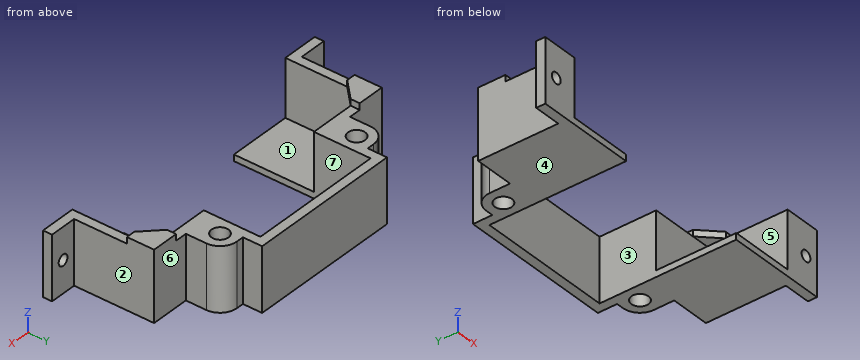
Autodesk Inventor part; units mm, degrees
ref_plane "YZ Plane" through (0, 0, 0) normal (1, 0, 0) x (0, 1, 0)
ref_plane "XZ Plane" through (0, 0, 0) normal (0, 1, 0) x (-1, 0, 0)
ref_plane "XY Plane" through (0, 0, 0) normal (0, 0, 1) x (1, 0, 0)
sketch "スケッチ1" plane through (0, 0, 0) normal (0, 0, 1) x (1, 0, 0)
  line L0 (0, 0) -> (0, 17.65)
  line L1 (0, 17.65) -> (28, 17.65)
  line L2 (28, 17.65) -> (28, 30.15)
  line L3 (28, 30.15) -> (58, 30.15)
  line L4 (58, 30.15) -> (58, 0)
  line L5 (58, 0) -> (60, 0)
  line L6 (60, 0) -> (60, 32.15)
  line L7 (60, 32.15) -> (28, 32.15)
  line L8 (28, 32.15) -> (26, 32.15)
  line L9 (26, 32.15) -> (26, 19.65)
  line L10 (26, 19.65) -> (-2, 19.65)
  line L11 (-2, 19.65) -> (-2, 0)
  line L12 (-2, 0) -> (0, 0)
  dimension "d0" = 17.65
  dimension "d1" = 28
  dimension "d2" = 12.5
  dimension "d3" = 30
  dimension "d4" = 2
  dimension "d5" = 32.15
  dimension "d6" = 32
  dimension "d7" = 2
  dimension "d8" = 12.5
  dimension "d9" = 28
extrude "押し出し1" add sketch "スケッチ1" along normal blind 14
sketch "スケッチ2" plane through (60, 0, 0) normal (1, 0, 0) x (0, 0, -1)
  line L0 (0, 0) -> (-14, 0)
  line L1 (-14, 0) -> (0, 0)
  line L2 (0, 0) -> (0, 2)
  line L3 (0, 2) -> (-14, 2)
  line L4 (-14, 2) -> (-14, 0)
  dimension "d12" = 14
  dimension "d13" = 2
extrude "押し出し2" add sketch "スケッチ2" along normal blind 7
sketch "スケッチ3" plane through (-2, 0, 0) normal (-1, 0, 0) x (0, 0, 1)
  line L0 (14, 2) -> (0, 2)
  line L1 (0, 0) -> (14, 0)
  line L2 (14, 0) -> (14, 2)
  line L3 (14, 2) -> (0, 2)
  line L4 (0, 2) -> (0, 0)
  dimension "d16" = 14
extrude "押し出し3" add sketch "スケッチ3" along normal blind 7
sketch "スケッチ4" plane through (0, 0, 14) normal (0, 0, 1) x (1, 0, 0)
  line L0 (60, 32.15) -> (60, 24.15)
  line L1 (60, 24.15) -> (61.6, 24.15)
  arc A0 (61.6, 20.4) -> (61.6, 27.9) centre (61.6, 24.15) ccw
  line L2 (61.6, 24.15) -> (61.6, 20.4) construction
  line L3 (61.6, 24.15) -> (61.6, 27.9) construction
  line L4 (61.6, 27.9) -> (60, 27.9)
  line L5 (61.6, 20.4) -> (60, 20.4)
  line L6 (60, 2) -> (60, 32.15)
  line L7 (60, 27.9) -> (60, 20.4)
  point P0 (0, 0)
  dimension "d47" = 8
  dimension "d48" = 1.6
  dimension "d49" = 3.75
  dimension "d50" = 180
extrude "押し出し4" add sketch "スケッチ4" against normal blind 14
hole "穴3" at (61.6, 24.15, 14) direction (0, 0, -1) diameter 3.75 end through all
sketch "スケッチ7" plane through (0, 0, 14) normal (0, 0, 1) x (1, 0, 0)
  line L0 (60, 32.15) -> (26, 32.15)
  line L1 (26, 32.15) -> (26, 24.15)
  line L2 (26, 24.15) -> (24.4, 24.15)
  arc A0 (24.4, 27.9) -> (24.4, 20.4) centre (24.4, 24.15) ccw
  line L3 (24.4, 27.9) -> (26, 27.9)
  line L4 (24.4, 20.4) -> (26, 20.4)
  line L5 (26, 20.4) -> (26, 27.9)
  line L6 (26, 32.15) -> (26, 19.65)
  circle A1 centre (24.4, 24.15) radius 1.875
  point P0 (0, 0)
  dimension "d60" = 8
  dimension "d61" = 1.6
  dimension "d62" = 3.75
  dimension "d63" = 3.75
extrude "押し出し6" add sketch "スケッチ7" against normal blind 14 contours L1 A1 L5 L4 A0 L3 | L1 L5 A1 picked at (23.6929, 24.15)
hole "穴4" at (24.4, 24.15, 14) direction (0, 0, -1) diameter 3.75 end through all
sketch "スケッチ10" plane through (0, 17.65, 0) normal (0, -1, 0) x (1, 0, 0)
  line L0 (28, 14) -> (58, 14)
  line L1 (0, 0) -> (28, 0)
  line L2 (28, 0) -> (28, 14)
  line L3 (28, 14) -> (0, 14)
  line L4 (0, 14) -> (0, 0)
extrude "押し出し7" cut sketch "スケッチ10" against normal blind 0.6
sketch "スケッチ11" plane through (0, 0, 0) normal (0, -1, 0) x (1, 0, 0)
  line L0 (0, 14) -> (-9, 14)
  line L1 (60, 0) -> (67, 0)
  line L2 (-9, 14) -> (67, 14)
  line L3 (67, 14) -> (67, 0)
  line L4 (67, 0) -> (-9, 0)
  line L5 (-9, 0) -> (-9, 14)
  point P0 (0, 0)
extrude "押し出し8" cut sketch "スケッチ11" against normal blind 0.6
sketch "スケッチ12" plane through (0, 0, 14) normal (0, 0, 1) x (1, 0, 0)
  line L0 (-2, 19.65) -> (-2, 2)
  line L1 (-2, 19.65) -> (4, 19.65)
  line L2 (26, 19.65) -> (-2, 19.65)
  line L3 (4, 19.65) -> (4, 18.25)
  line L4 (0, 18.25) -> (28, 18.25)
  line L5 (4, 18.25) -> (0.2844, 14.5344)
  line L6 (4, 18.25) -> (9.2547, 18.25) construction
  line L7 (0.2844, 14.5344) -> (0, 14.25)
  line L8 (0, 0.6) -> (0, 18.25)
  line L9 (0, 14.25) -> (-2, 14.25)
  line L10 (-2, 14.25) -> (-2, 19.65)
  point P0 (0, 0)
  dimension "d79" = 6
  dimension "d80" = 135
extrude "押し出し9" add sketch "スケッチ12" along normal blind 2
sketch "スケッチ15" plane through (0, 0, 0) normal (0, 0, -1) x (-1, 0, 0)
  line L0 (0, 0.6) -> (0, 18.25)
  line L1 (0, 18.25) -> (-14, 18.25)
  line L2 (-14, 18.25) -> (-14, 0.6)
  line L3 (-14, 0.6) -> (0, 0.6)
  line L4 (0, 0.6) -> (0, 18.25)
  point P0 (0, 0)
  dimension "d88" = 14
extrude "押し出し11" add sketch "スケッチ15" against normal blind 1.4
sketch "スケッチ17" plane through (67, 0, 0) normal (1, 0, 0) x (0, 0, -1)
  line L0 (0, 0.6) -> (-14, 0.6)
  line L1 (0, 0.6) -> (-14, 0.6)
  line L2 (-14, 0.6) -> (-14, 9.5309)
  line L3 (-14, 9.5309) -> (0, 9.5309)
  line L4 (0, 9.5309) -> (0, 0.6)
  point P0 (0, 0)
extrude "押し出し13" cut sketch "スケッチ17" against normal blind 3
sketch "スケッチ18" plane through (-9, 0, 0) normal (-1, 0, 0) x (0, 0, 1)
  line L0 (0, 0.6) -> (14, 0.6)
  line L1 (0, 0.6) -> (14, 0.6)
  line L2 (14, 0.6) -> (14, 6.5)
  line L3 (14, 6.5) -> (0, 6.5)
  line L4 (0, 6.5) -> (0, 0.6)
  point P0 (0, 0)
extrude "押し出し14" cut sketch "スケッチ18" against normal blind 3
hole "穴5" at (-4, 2, 7) direction (0, -1, 0) diameter 2.4 end through all
hole "穴6" at (62, 2, 7) direction (0, -1, 0) diameter 2.4 end through all
mirror "ミラー1" about plane through (31.8158, 20.0509, 0) normal (0, 0, -1) of "押し出し3", "押し出し1", "押し出し4", "穴3", "押し出し2", "穴6", "穴4", "押し出し6", "押し出し7", "押し出し9", "押し出し11", "押し出し14", "押し出し13", "穴5", "押し出し8"
sketch "スケッチ19" plane through (0, 0, 14) normal (0, 0, 1) x (1, 0, 0)
  line L0 (94.8832, 81.412) -> (-62.365, 81.412)
  line L1 (-62.365, 81.412) -> (-62.365, -71.7744)
  line L2 (-62.365, -71.7744) -> (94.8832, -71.7744)
  line L3 (94.8832, -71.7744) -> (94.8832, 81.412)
  point P0 (0, 0)
extrude "押し出し15" cut sketch "スケッチ19" against normal blind 14
sketch "スケッチ20" plane through (-2, 19.65, 14) normal (0, 1, 0) x (1, 0, 0)
  line L0 (17.6833, -4.2941) -> (-12.6138, -4.2941)
  line L1 (-12.6138, -4.2941) -> (-12.6138, 1.0873)
  line L2 (-12.6138, 1.0873) -> (17.6833, 1.0873)
  line L3 (17.6833, 1.0873) -> (17.6833, -4.2941)
  point P0 (2, 14)
extrude "押し出し16" cut sketch "スケッチ20" against normal blind 14
sketch "スケッチ21" plane through (26, 27.9, -14) normal (-1, 0, 0) x (0, 0, 1)
  line L0 (0, -8.25) -> (-2, -8.25)
  line L1 (-2, -8.25) -> (18.9234, -8.25)
  line L2 (18.9234, -8.25) -> (18.9234, 5.2405)
  line L3 (18.9234, 5.2405) -> (-2, 5.2405)
  line L4 (-2, 5.2405) -> (-2, -8.25)
  point P0 (14, -27.9)
split body "分割1" sketch "スケッチ21" result one side removed curves L2 L3 L4 L1 removed pieces at (9.3333, 19.15, -4.6667) (58.5, 13.3, -4.6667)
sketch "スケッチ22" plane through (0, 0, 0) normal (0, 0, 1) x (1, 0, 0)
  line L0 (28, 19.65) -> (28, 30.15)
  line L1 (28, 19.65) -> (28, 17.65)
  line L2 (28, 17.65) -> (14, 17.65)
  line L3 (14, 17.65) -> (14, 0)
  line L4 (14, 17.65) -> (31.65, 17.65) construction
  line L5 (14, 0) -> (8, 0)
  line L6 (8, 0) -> (8, 2)
  line L7 (8, 2) -> (12, 2)
  line L8 (26.0798, 19.65) -> (12, 19.65)
  line L9 (12, 19.65) -> (12, 2)
  line L10 (58, 19.65) -> (60, 19.65)
  line L11 (58, 19.65) -> (58, 17.65)
  line L12 (58, 17.65) -> (72, 17.65)
  line L13 (72, 17.65) -> (72, 0)
  line L14 (72, 0) -> (78, 0)
  line L15 (78, 0) -> (78, 2)
  line L16 (78, 2) -> (74, 2)
  line L17 (74, 2) -> (74, 19.65)
  line L18 (74, 19.65) -> (60, 19.65)
  line L19 (26.0798, 19.65) -> (28, 19.65)
  line L20 (24.4, 20.4) -> (26, 20.4)
  line L21 (58, 19.65) -> (60, 19.65)
  point P0 (0, 0)
  dimension "d119" = 2
  dimension "d120" = 14
  dimension "d121" = 17.65
  dimension "d122" = 90
  dimension "d123" = 6
  dimension "d124" = 2
  dimension "d125" = 4
  dimension "d126" = 14
  dimension "d127" = 6
  dimension "d128" = 2
  dimension "d129" = 4
extrude "押し出し17" add sketch "スケッチ22" against normal blind 14
sketch "スケッチ23" plane through (26, 32.15, -14) normal (0, 1, 0) x (1, 0, 0)
  line L0 (32, -14) -> (2, -14)
  line L1 (17, -14) -> (17, 0)
  line L2 (2, 0) -> (32, 0)
  point P0 (-26, -14)
sketch "スケッチ25" plane through (24.4, 24.15, -14) normal (0, 0, -1) x (-1, 0, 0)
  line L0 (-3.6, -6.5) -> (10.4, -6.5)
  line L1 (10.4, -6.5) -> (-3.6, -6.5)
  line L2 (-3.6, -6.5) -> (-3.6, -24.15)
  line L3 (-3.6, -24.15) -> (10.4, -24.15)
  line L4 (10.4, -24.15) -> (10.4, -6.5)
  point P0 (24.4, -24.15)
extrude "押し出し18" add sketch "スケッチ25" against normal blind 1.4
ref_plane "作業平面1" through (43, 32.15, 0) normal (1, 0, 0) x (0, 0, -1)
mirror "ミラー3" about plane through (43, 32.15, 0) normal (1, 0, 0) of "押し出し18"
sketch "スケッチ26" plane through (0, 0, 0) normal (0, 0, 1) x (1, 0, 0)
  line L0 (12, 2) -> (12, 19.65)
  line L1 (12, 19.65) -> (18, 19.65)
  line L2 (12, 19.65) -> (26, 19.65)
  line L3 (18, 19.65) -> (18, 17.65)
  line L4 (28, 17.65) -> (14, 17.65)
  line L5 (18, 17.65) -> (14, 13.65)
  line L6 (14, 17.65) -> (14, 0)
  line L7 (18, 17.65) -> (23.6569, 17.65) construction
  line L8 (14, 13.65) -> (12, 13.65)
  line L9 (12, 13.65) -> (12, 19.65)
  point P0 (0, 0)
  dimension "d139" = 6
  dimension "d140" = 135
extrude "押し出し20" add sketch "スケッチ26" along normal blind 1.4
mirror "ミラー4" about plane through (43, 32.15, 0) normal (1, 0, 0) of "押し出し20"
sketch "スケッチ27" plane through (0, 0, 0) normal (0, 0, 1) x (1, 0, 0)
  line L0 (8, 2) -> (12, 2)
  line L1 (8, 2) -> (6, 2)
  line L2 (6, 2) -> (6, 0)
  line L3 (6, 0) -> (8, 0)
  line L4 (8, 0) -> (8, 2)
  line L5 (78, 2) -> (80, 2)
  line L6 (80, 2) -> (80, 0)
  line L7 (80, 0) -> (78, 0)
  line L8 (78, 0) -> (78, 2)
  point P0 (0, 0)
  dimension "d143" = 2
  dimension "d144" = 2
extrude "押し出し21" add sketch "スケッチ27" against normal blind 14
hole "穴7" at (77, 2, -7) direction (0, -1, 0) diameter 2.4 end through all
hole "穴8" at (9, 2, -7) direction (0, -1, 0) diameter 2.4 end through all
sketch "スケッチ28" plane through (0, 0, 0) normal (0, 0, 1) x (1, 0, 0)
  arc A0 (24.4, 27.9) -> (24.4, 20.4) centre (24.4, 24.15) ccw
  line L0 (20.65, 24.15) -> (20.65, 19.65)
  line L1 (12, 19.65) -> (26, 19.65)
  line L2 (24.4, 20.4) -> (26, 20.4)
  line L3 (26, 19.65) -> (26, 20.4)
  line L4 (26, 20.4) -> (20.65, 24.15)
  point P0 (0, 0)
extrude "押し出し22" add sketch "スケッチ28" against normal blind 14 contours A0 L2 L3 L1 L0
mirror "ミラー5" about plane through (43, 32.15, 0) normal (1, 0, 0) of "押し出し22"
properties part number "センサ冶具1セット"
Geometry: final body of the model. Coordinates: model frame, mm. Face numbers are marked on the shaded views. A direction names the side the tool comes from. Coordinates: 2 decimals unless noted, no trailing zeros. Loops run counter-clockwise (first coordinate to the right, second up) from the corner with the lowest first, then second, coordinate; pieces in that order, holes last. Notation, with made-up numbers: (55, 15) -> (111, 15) arc R20 ccw to (111, 49) -> close; hole circle Ø11 at (-38.5, -8.75). An arc over 180 degrees is marked (long way). Use a Markdown table: item, result. Add a question column.
(1) Section query D-D, the plane x = 17. Return loops of the section in (y, z), plus the area to 3 significant figures.
(2) Section query C-C, the plane z = -10. Return loops of the section in (x, y) (3 decimals).
(3) Section query B-B, the plane x = 77. Return loops of the section in (y, z).
(4) Access query for the marked faces 5, 6 and 7. Directions: +Z, -Z, +X, -X, +Y, -Y. A direction counts if a zero-diameter tool reaches every point of the face in a straight line with its end or side. Return the directions, or none.
(5) Section query A-A, the plane y = 20.5. Return loops of the section in (x, z).
(6) Mould query, pull axis X, two halves, no side actions, for the marked faces 1, 2, 3 and 4. Classes: pulls with the +X half, pulls with the -X half, needs draft (parallel to the pull), parting line crosses it, or undercut.
(7) Pin query (flat end, axial travel): pin 1 Ø11.5 at (x, y) = (40, 27.5) entering from +Z; pin 2 Ø6.5 at (x, z) = (76.5, -9) entering from +Y; pin 3 Ø3 at (x, z) = (56, -12) entering from -Y. Return the tip coordinate at first contact, or that it passes through.
(8) Line query: line 1 along X through (y, z) = (24.15, -3.5) (3 decimals); line 2 along X through (y, z) = (1, -7); line 3 along Y through (x, z) = (24.4, -4.5) (3 decimals). Output: solid intervals per line, ascending.
Answer:
| question | item | result |
|---|---|---|
| 1 | outline | (0, -14) -> (19.65, -14) -> (19.65, 1.4) -> (16.65, 1.4) -> (16.65, 0) -> (17.65, 0) -> (17.65, -12.6) -> (0, -12.6) -> close |
| 1 | area | 56.9 mm^2 |
| 2 | outline | (6, 0) -> (14, 0) -> (14, 17.65) -> (28, 17.65) -> (28, 30.15) -> (58, 30.15) -> (58, 17.65) -> (72, 17.65) -> (72, 0) -> (80, 0) -> (80, 2) -> (74, 2) -> (74, 19.65) -> (65.35, 19.65) -> (65.35, 24.15) arc R3.75 ccw to (61.6, 27.9) -> (60, 27.9) -> (60, 32.15) -> (26, 32.15) -> (26, 27.9) -> (24.4, 27.9) arc R3.75 ccw to (20.65, 24.15) -> (20.65, 19.65) -> (12, 19.65) -> (12, 2) -> (6, 2) -> close; hole circle Ø3.75 at (24.4, 24.15); hole circle Ø3.75 at (61.6, 24.15) |
| 3 | outline | (0, -14) -> (2, -14) -> (2, -8.2) -> (0, -8.2) -> close; (0, -5.8) -> (2, -5.8) -> (2, 0) -> (0, 0) -> close |
| 4 | face 5 | -Y |
| 4 | face 6 | +Z, -Z, +X, +Y |
| 4 | face 7 | +Z, -Z, -Y |
| 5 | outline | (20.65, -14) -> (28, -14) -> (28, 0) -> (20.65, 0) -> close; (58, -14) -> (65.35, -14) -> (65.35, 0) -> (58, 0) -> close |
| 6 | face 1 | undercut |
| 6 | face 2 | pulls with the +X half |
| 6 | face 3 | undercut |
| 6 | face 4 | needs draft |
| 7 | pin 1 | stops at z = 0 |
| 7 | pin 2 | stops at y = 19.65 |
| 7 | pin 3 | stops at y = 30.15 |
| 8 | line 1 | x = 20.65 to 22.525, 26.275 to 28, 58 to 59.725, 63.475 to 65.35 |
| 8 | line 2 | x = 6 to 7.8, 10.2 to 14, 72 to 75.8, 78.2 to 80 |
| 8 | line 3 | y = 17.65 to 22.275, 26.025 to 27.9 |
